Study the drawing (mm; zero at the part's minimum x, y, z) and answer. A direction names the side the tool comes from. Give positions to 0.01 mm unless a question says otherwise; leave off trailing zeros. Write each loop counter-clockwise with the first axis right and the second up, starting at its lowest first coordinate (ties: lowest second). Pieces come first, ordered by that corner, then holes. Notation, with made-up numbers: (82, 15) - (136, 15) arc R27 cw to (136, 36) - close; hole circle Ø5 at (15.5, -38.75). An arc over 180 degrees is marked (long way). Answer as CSV lines item,"result".
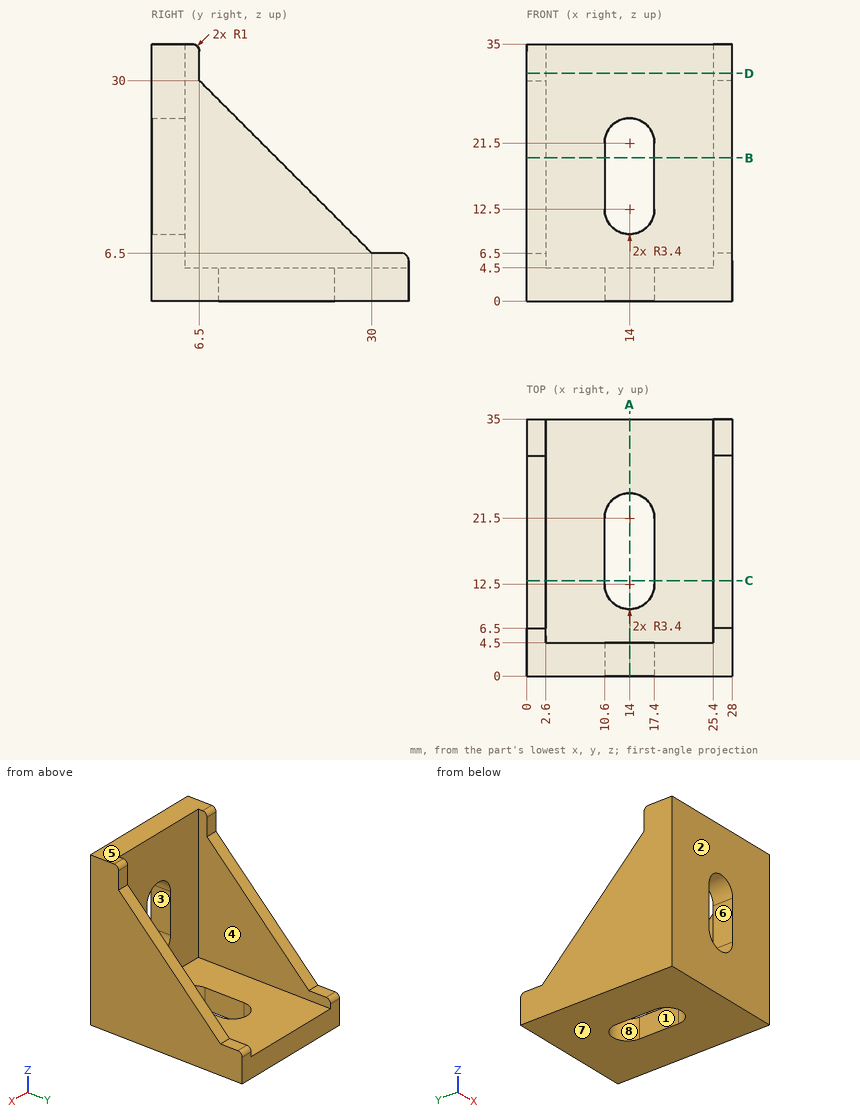
(1) A cutting plane is placed at D-D (z = 31). Write down the section's boundary in (x, y), and give its area (3 significant figures).
Worked out:
outline,"(0, 0) - (28, 0) - (28, 6.5) - (25.4, 6.5) - (25.4, 4.5) - (2.6, 4.5) - (2.6, 6.5) - (0, 6.5) - close"
area,"136 mm^2"
(2) For the marked faces 1, 2, 3 and 4, determine the directions among +Z, -Z, +X, -X, +Y, -Y from which every point of the face is accessible in a straight line to the end or side of a thin tool.
Worked out:
face 1,"+Z, -Z"
face 2,"+Z, -Z, +X, -X, -Y"
face 3,"+Y, -Y"
face 4,"+Z, +Y"
(3) A cutting plane is placed at A-A (x = 14). Write down the section's boundary in (y, z), and give its area (3 significant figures).
Worked out:
outline,"(0, 0) - (9.1, 0) - (9.1, 4.5) - (4.5, 4.5) - (4.5, 9.1) - (0, 9.1) - close; (0, 24.9) - (4.5, 24.9) - (4.5, 35) - (0, 35) - close; (24.9, 0) - (35, 0) - (35, 4.5) - (24.9, 4.5) - close"
area,"153 mm^2"
(4) A cutting plane is placed at B-B (z = 19.5). Write down the section's boundary in (x, y).
Worked out:
outline,"(0, 0) - (10.6, 0) - (10.6, 4.5) - (2.6, 4.5) - (2.6, 17) - (0, 17) - close; (17.4, 0) - (28, 0) - (28, 17) - (25.4, 17) - (25.4, 4.5) - (17.4, 4.5) - close"
(5) A cutting plane is placed at C-C (y = 13). Write down the section's boundary in (x, z), and give its area (3 significant figures).
Worked out:
outline,"(0, 0) - (10.6, 0) - (10.6, 4.5) - (2.6, 4.5) - (2.6, 23.5) - (0, 23.5) - close; (17.4, 0) - (28, 0) - (28, 23.5) - (25.4, 23.5) - (25.4, 4.5) - (17.4, 4.5) - close"
area,"194 mm^2"
(6) Each of these flat-tipped pins is pushed along its axis until it touches: P1, Ø7, axis at x = 13, y = 19.5, coming from the +Z side; P2, Ø11.5, axis at x = 10.5, z = 14, coming from the +Y side; P3, Ø2, axis at x = 1.5, z = 32.5, coming from the +Y side; P4, Ø6, axis at y = 24.5, z = 17, coming from the -X side. Where does it stop, or does it pass through?
Worked out:
P1,"stops at z = 4.5"
P2,"stops at y = 4.5"
P3,"stops at y = 6.5"
P4,"passes through"
(7) Find the intervals of material crossed by L1, parallel to X at y = 7.5, z = 16.5; L2, parallel to Z at x = 19.25, y = 32.5, in increasing order.
Worked out:
L1,"x = 0 to 2.6, 25.4 to 28"
L2,"z = 0 to 4.5"
(8) The mould has two halves that part along Z. Classify the marked faces 5, 6, 7 and 8: +Z half, -Z half, draft (parallel to the pull), parting line (faces both ways), or undercut.
Worked out:
face 5,"+Z half"
face 6,"undercut"
face 7,"-Z half"
face 8,"draft"
